The listing builds one solid part. Answer for the finished solid, in the listing's coordinates (mm). A direction names the side the tool comes from. Give positions to 0.01 mm unless a question says otherwise; leave off trailing zeros. Write each loop counter-clockwise with the first axis right and the second up, starting at its lowest first coordinate (ties: lowest second). Pieces come first, ordered by that corner, then holes. Notation, with made-up numbers: (-27, 45.25) - (4, 45.25) arc R15 cw to (4, 63.25) - close; hole circle Ø10 at (35, 30.25). An arc over 180 degrees is marked (long way). Write each question's results on one line, items separated by ' | '. Start each with the question number.
Q1. Section C-C (y = -46) is taken. Determine the outline of the cut face in (x, z), plus the area to 3 significant figures.
Q2. Flat-ended cylindrical pins translate along their axes: pin 1 Ø3 at (x, z) = (-21, 17.5) entering from +Y; pin 2 Ø12 at (x, y) = (-24, -47) entering from -Z; pin 3 Ø4 at (x, z) = (-64.5, 17) entering from -Y; pin 4 Ø10 at (y, z) = (-45.5, 26.5) entering from +X. Find the tip coordinate at first contact, or state that the pin passes through.
Q3. Find the intervals of material crossed by probe 1 along Y at (x, z) = (-49, 15); probe 2 along X at (y, z) = (-34.5, 4); probe 3 along X at (y, z) = (-23, 6), in increasing order.
Q4. Section D-D (x = -49.5) is taken. Determine the outline of the cut face in (y, z), plus the area to 3 significant figures.
Q5. For faces 1 (the face through (-91.661, -35, 16)), 2 (the face through (-40, -41.999, 16)), 3 (the face through (-37, -29.299, 16)), determine the directions among +Z, -Z, +X, -X, +Y, -Y from which every point of the face is accessible in a straight line to the end or side of a thin tool.
Q6. Section A-A (z = 19) is taken. Determine the outline of the cut face in (x, y).
Q7. Section B-B (x = -63) is taken. Determine the outline of the cut face in (y, z), plus the area to 3 significant figures.
```python
from build123d import *

# Parameters (mm, degrees)
F1_DEPTH = 31.75
F3_DEPTH = 25.4
F5_DEPTH = 12.7
F7_DEPTH = 12.7
F9_DEPTH = 12.7


# Not quite as in the source:
# - a length typed as a fraction of an inch, garbled in the dataset ("3 / 203.2 mm" for 3/8 in), is restored


with BuildPart() as f1:
    # F0 (on Top) → F1 (new body)
    with BuildSketch(Plane.XY):
        Polygon((-59.9109128669, -16.5989177401), (-91.6609128669, -16.5989177401), (-91.6609128669, -54.6989177401), (-59.9109128669, -54.6989177401), (-59.9109128669, -41.9989177401), (-2.7609128669, -41.9989177401), (-2.7609128669, -29.2989177401), (-59.9109128669, -29.2989177401), align=None)
    extrude(amount=F1_DEPTH)

    # F2 (on face) → F3 (cut)
    with BuildSketch(Plane.XZ.offset(54.6989177401)):
        Polygon((-74.4201987982, 31.75), (-59.9109128669, 0), (-59.9109128669, 31.75), align=None)
    extrude(amount=F3_DEPTH, mode=Mode.SUBTRACT)

    # F4 (on face) → F5 (cut)
    with BuildSketch(Plane.XZ.offset(54.6989177401)):
        Polygon((-75.7859128669, 31.75), (-59.9109128669, 0), (-46.3341996074, 12.059702538), (-46.3341996074, 45.9536202252), (-62.0433166623, 45.9536202252), align=None)
    extrude(amount=-F5_DEPTH, mode=Mode.SUBTRACT)

    # F6 (on face) → F7 (cut)
    with BuildSketch(Plane(origin=(0, -16.5989177401, 0), x_dir=(-1, 0, 0), z_dir=(0, 1, 0))):
        Polygon((59.9109128669, 0), (72.6109128669, 31.75), (59.9109128669, 31.75), align=None)
    extrude(amount=-F7_DEPTH, mode=Mode.SUBTRACT)

    # F8 (on face) → F9 (cut)
    with BuildSketch(Plane.XZ.offset(41.9989177401)):
        Polygon((-15.4609128669, 31.75), (-2.7609128669, 0), (-2.7609128669, 31.75), align=None)
    extrude(amount=-F9_DEPTH, mode=Mode.SUBTRACT)


solid = f1.part
```
Answers below:
1) outline: (-91.66, 0) - (-59.91, 0) - (-75.79, 31.75) - (-91.66, 31.75) - close | area: 756 mm2
2) pin 1: stops at y = -29.3 | pin 2: stops at z = 0 | pin 3: stops at y = -42 | pin 4: stops at x = -11.93
3) probe 1: y = -42 to -29.3 | probe 2: x = -91.66 to -4.36 | probe 3: x = -91.66 to -62.31
4) outline: (-42, 0) - (-29.3, 0) - (-29.3, 31.75) - (-42, 31.75) - close | area: 403 mm2
5) face 1: +Z, -Z, -X, +Y, -Y | face 2: +Z, +X, -Y | face 3: +Z, +X, +Y
6) outline: (-91.66, -54.7) - (-69.41, -54.7) - (-69.41, -42) - (-10.36, -42) - (-10.36, -29.3) - (-67.51, -29.3) - (-67.51, -16.6) - (-91.66, -16.6) - close
7) outline: (-54.7, 0) - (-16.6, 0) - (-16.6, 7.72) - (-29.3, 7.72) - (-29.3, 31.75) - (-42, 31.75) - (-42, 6.18) - (-54.7, 6.18) - close | area: 580 mm2
